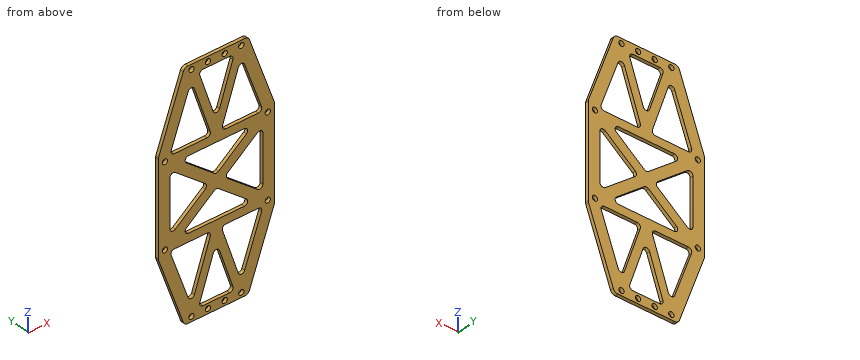
from build123d import *

# Parameters (mm, degrees)
SKETCH_1_R          = 1.6
EXTRUDE_1_DEPTH     = 2
CUT_EXTRUDE_1_DEPTH = 3
FILLET_1_R          = 3


with BuildPart() as part:
    # 草图1 → 凸台-拉伸1 (new body)
    with BuildSketch(Plane(origin=(0, 0, 0), x_dir=(1, 0, 0), z_dir=(0, 1, 0))):
        Polygon((35, -28.67494242), (19.239979527, -73), (-19.239979527, -73), (-35, -28.67494242), (-35, 28.67494242), (-19.239979527, 73), (19.239979527, 73), (35, 28.67494242), align=None)
        with Locations((-31, 25)):
            Circle(SKETCH_1_R, mode=Mode.SUBTRACT)
        with Locations((-31, -25)):
            Circle(SKETCH_1_R, mode=Mode.SUBTRACT)
        with Locations((31, -25)):
            Circle(SKETCH_1_R, mode=Mode.SUBTRACT)
        with Locations((31, 25)):
            Circle(SKETCH_1_R, mode=Mode.SUBTRACT)
        with Locations((-15, 70)):
            Circle(SKETCH_1_R, mode=Mode.SUBTRACT)
        with Locations((-5, 70)):
            Circle(SKETCH_1_R, mode=Mode.SUBTRACT)
        with Locations((5, 70)):
            Circle(SKETCH_1_R, mode=Mode.SUBTRACT)
        with Locations((15, 70)):
            Circle(SKETCH_1_R, mode=Mode.SUBTRACT)
        with Locations((-5, -70)):
            Circle(SKETCH_1_R, mode=Mode.SUBTRACT)
        with Locations((5, -70)):
            Circle(SKETCH_1_R, mode=Mode.SUBTRACT)
        with Locations((15, -70)):
            Circle(SKETCH_1_R, mode=Mode.SUBTRACT)
        with Locations((-15, -70)):
            Circle(SKETCH_1_R, mode=Mode.SUBTRACT)
    extrude(amount=EXTRUDE_1_DEPTH)

    # 草图2 → 切除-拉伸1 (cut, through all)
    with BuildSketch(Plane(origin=(0, 2, 0), x_dir=(1, 0, 0), z_dir=(0, 1, 0))):
        with BuildLine():
            Line((-3.652336951, -29.632455532), (-13.224638858, -58.349361255))
            ThreePointArc((-13.224638858, -58.349361255), (-15.102140845, -59.71680707), (-17.006434835, -58.386925058))
            Line((-17.006434835, -58.386925058), (-27.216890203, -29.670019335))
            ThreePointArc((-27.216890203, -29.670019335), (-26.966480203, -27.846752123), (-25.332460823, -27))
            Line((-25.332460823, -27), (-5.549703547, -27))
            ThreePointArc((-5.549703547, -27), (-3.927219177, -27.830579431), (-3.652336951, -29.632455532))
        make_face()
        with BuildLine():
            Line((-1.897366596, -40.178932769), (-9.960237162, -64.367544468))
            ThreePointArc((-9.960237162, -64.367544468), (-9.685354937, -66.169420569), (-8.062870566, -67))
            Line((-8.062870566, -67), (8.062870566, -67))
            ThreePointArc((8.062870566, -67), (9.685354937, -66.169420569), (9.960237162, -64.367544468))
            Line((9.960237162, -64.367544468), (1.897366596, -40.178932769))
            ThreePointArc((1.897366596, -40.178932769), (0, -38.811388301), (-1.897366596, -40.178932769))
        make_face()
        with BuildLine():
            Line((5.549703547, -27), (25.332460823, -27))
            ThreePointArc((25.332460823, -27), (26.966480203, -27.846752123), (27.216890203, -29.670019335))
            Line((27.216890203, -29.670019335), (17.006434835, -58.386925058))
            ThreePointArc((17.006434835, -58.386925058), (15.102140845, -59.71680707), (13.224638858, -58.349361255))
            Line((13.224638858, -58.349361255), (3.652336951, -29.632455532))
            ThreePointArc((3.652336951, -29.632455532), (3.927219177, -27.830579431), (5.549703547, -27))
        make_face()
        with BuildLine():
            Line((-28, 14.544416854), (-28, -14.544416854))
            ThreePointArc((-28, -14.544416854), (-26.862841293, -16.348718631), (-24.744495098, -16.101242933))
            Line((-24.744495098, -16.101242933), (-6.709418198, -1.556826079))
            ThreePointArc((-6.709418198, -1.556826079), (-5.964923101, 0), (-6.709418198, 1.556826079))
            Line((-6.709418198, 1.556826079), (-24.744495098, 16.101242933))
            ThreePointArc((-24.744495098, 16.101242933), (-26.862841293, 16.348718631), (-28, 14.544416854))
        make_face()
        with BuildLine():
            Line((24.744495098, -16.101242933), (6.709418198, -1.556826079))
            ThreePointArc((6.709418198, -1.556826079), (5.964923101, 0), (6.709418198, 1.556826079))
            Line((6.709418198, 1.556826079), (24.744495098, 16.101242933))
            ThreePointArc((24.744495098, 16.101242933), (26.862841293, 16.348718631), (28, 14.544416854))
            Line((28, 14.544416854), (28, -14.544416854))
            ThreePointArc((28, -14.544416854), (26.862841293, -16.348718631), (24.744495098, -16.101242933))
        make_face()
        with BuildLine():
            Line((-18.090581802, -18.443173921), (-1.255504902, -4.866499002))
            ThreePointArc((-1.255504902, -4.866499002), (0, -4.423325081), (1.255504902, -4.866499002))
            Line((1.255504902, -4.866499002), (18.090581802, -18.443173921))
            ThreePointArc((18.090581802, -18.443173921), (18.721031851, -20.665713092), (16.835076899, -22))
            Line((16.835076899, -22), (0, -22))
            Line((0, -22), (-16.835076899, -22))
            ThreePointArc((-16.835076899, -22), (-18.721031851, -20.665713092), (-18.090581802, -18.443173921))
        make_face()
        with BuildLine():
            Line((-16.835076899, 22), (0, 22))
            Line((0, 22), (16.835076899, 22))
            ThreePointArc((16.835076899, 22), (18.721031851, 20.665713092), (18.090581802, 18.443173921))
            Line((18.090581802, 18.443173921), (1.255504902, 4.866499002))
            ThreePointArc((1.255504902, 4.866499002), (0, 4.423325081), (-1.255504902, 4.866499002))
            Line((-1.255504902, 4.866499002), (-18.090581802, 18.443173921))
            ThreePointArc((-18.090581802, 18.443173921), (-18.721031851, 20.665713092), (-16.835076899, 22))
        make_face()
        with BuildLine():
            Line((9.960237162, 64.367544468), (1.897366596, 40.178932769))
            ThreePointArc((1.897366596, 40.178932769), (0, 38.811388301), (-1.897366596, 40.178932769))
            Line((-1.897366596, 40.178932769), (-9.960237162, 64.367544468))
            ThreePointArc((-9.960237162, 64.367544468), (-9.685354937, 66.169420569), (-8.062870566, 67))
            Line((-8.062870566, 67), (8.062870566, 67))
            ThreePointArc((8.062870566, 67), (9.685354937, 66.169420569), (9.960237162, 64.367544468))
        make_face()
        with BuildLine():
            Line((13.224638858, 58.349361255), (3.652336951, 29.632455532))
            ThreePointArc((3.652336951, 29.632455532), (3.927219177, 27.830579431), (5.549703547, 27))
            Line((5.549703547, 27), (25.332460823, 27))
            ThreePointArc((25.332460823, 27), (26.966480203, 27.846752123), (27.216890203, 29.670019335))
            Line((27.216890203, 29.670019335), (17.006434835, 58.386925058))
            ThreePointArc((17.006434835, 58.386925058), (15.102140845, 59.71680707), (13.224638858, 58.349361255))
        make_face()
        with BuildLine():
            Line((-25.332460823, 27), (-5.549703547, 27))
            ThreePointArc((-5.549703547, 27), (-3.927219177, 27.830579431), (-3.652336951, 29.632455532))
            Line((-3.652336951, 29.632455532), (-13.224638858, 58.349361255))
            ThreePointArc((-13.224638858, 58.349361255), (-15.102140845, 59.71680707), (-17.006434835, 58.386925058))
            Line((-17.006434835, 58.386925058), (-27.216890203, 29.670019335))
            ThreePointArc((-27.216890203, 29.670019335), (-26.966480203, 27.846752123), (-25.332460823, 27))
        make_face()
    extrude(amount=-CUT_EXTRUDE_1_DEPTH, mode=Mode.SUBTRACT)

    # 圆角1
    fillet_1_edges = [part.edges().sort_by_distance(p)[0] for p in [
        (35, 1, 28.67494242),
        (19.239979527, 1, 73),
        (-19.239979527, 1, 73),
        (-35, 1, 28.67494242),
        (-35, 1, -28.67494242),
        (-19.239979527, 1, -73),
        (19.239979527, 1, -73),
        (35, 1, -28.67494242),
    ]]
    fillet(fillet_1_edges, radius=FILLET_1_R)


solid = part.part
Part model, mm, in its own coordinate system. Coordinates: 2 decimals unless noted, no trailing zeros. Order: outer loops, then holes, each group sorted by start corner. A loop starts at its lowest first (then second) coordinate and runs counter-clockwise, first axis right, second up. Notation, with made-up numbers: M 76.5,33 L 93.5,33 A29 cw 93.5,60 Z; hole C 39.5,88 d1. An arc over 180 degrees is marked long. One line per question, with ' | ' between items.
Q1. Slice it at A-A (z = -25). Give the cut face in (x, y).
A:
outline: M -35,0 L -32.6,0 L -32.6,2 L -35,2 Z; M -29.4,0 L 29.4,0 L 29.4,2 L -29.4,2 Z; M 32.6,0 L 35,0 L 35,2 L 32.6,2 Z
Q2. Slice it at B-B (x = 31). Give the cut face in (y, z), and give its area (3 significant figures).
A:
outline: M 0,-39.92 L 2,-39.92 L 2,-26.6 L 0,-26.6 Z; M 0,-23.4 L 2,-23.4 L 2,23.4 L 0,23.4 Z; M 0,26.6 L 2,26.6 L 2,39.92 L 0,39.92 Z | area: 147 mm^2
Q3. Slice it at C-C (y = 1.55). Count the separate pieces of the cut face and the enclosed holes in it, and give its area (3 significant figures).
A:
separate pieces: 1 | enclosed holes: 22 | area: 4,570 mm^2
Q4. Drill centre lines: line 1 (X direction, y = 1.3, z = -25); line 2 (X direction, y = 1.6, z = 51.5); line 3 (X direction, y = 0.8, z = 11). Where is each one in solid material? Low to high.
A:
line 1: x = -35 to -32.6, -29.4 to 29.4, 32.6 to 35 | line 2: x = -26.88 to -19.46, -10.94 to -5.67, 5.67 to 10.94, 19.46 to 26.88 | line 3: x = -35 to -28, -18.42 to -8.86, 8.86 to 18.42, 28 to 35
Q5. Slice it at D-D (z = -53.5). Give the cut face in (x, y).
A:
outline: M -26.17,0 L -18.74,0 L -18.74,2 L -26.17,2 Z; M -11.61,0 L -6.34,0 L -6.34,2 L -11.61,2 Z; M 6.34,0 L 11.61,0 L 11.61,2 L 6.34,2 Z; M 18.74,0 L 26.17,0 L 26.17,2 L 18.74,2 Z
Q6. Pin check, flat tips, straight feed: P1, Ø4, axis at x = -5, z = 70, coming from the +Y side; P2, Ø1, axis at x = -20, y = 1, coming from the -Z side; P3, Ø1, axis at y = 1.5, z = 35, coming from the +X side. Stop position of each tip, or through.
A:
P1: stops at y = 2 | P2: stops at z = -71.83 | P3: stops at x = 32.93
